Autodesk Inventor part; units mm, degrees
ref_plane "YZ Plane" through (0, 0, 0) normal (1, 0, 0) x (0, 1, 0)
ref_plane "XZ Plane" through (0, 0, 0) normal (0, 1, 0) x (-1, 0, 0)
ref_plane "XY Plane" through (0, 0, 0) normal (0, 0, 1) x (1, 0, 0)
sketch "Sketch1" plane through (0, 0, 0) normal (0, 0, 1) x (1, 0, 0)
  line L0 (6.35, 0) -> (25.4, 0)
  line L1 (25.4, 0) -> (25.4, -3.175)
  line L2 (25.4, -3.175) -> (6.35, -3.175)
  line L3 (3.175, -6.35) -> (3.175, -38.1)
  line L4 (3.175, -38.1) -> (0, -38.1)
  line L5 (0, -38.1) -> (0, -6.35)
  arc A0 (6.35, -3.175) -> (3.175, -6.35) centre (6.35, -6.35) ccw
  arc A1 (6.35, 0) -> (0, -6.35) centre (6.35, -6.35) ccw
  point P0 (0, 0)
  dimension "d0" = 3.175
  dimension "d1" = 38.1
  dimension "d2" = 3.175
  dimension "d3" = 6.35
  dimension "d6" = 25.4
extrude "Extrusion1" add sketch "Sketch1" along normal blind 50.8
hole "Hole1" at (12.7, -3.175, 38.1) direction (0, 1, 0) diameter 4.826 depth 25.4 tip angle 118
pattern_linear "Rectangular Pattern1" count 2 spacing 25 along (0, 0, -1) of "Hole1"
hole "Hole2" at (3.175, -19.05, 38.1) direction (-1, 0, 0) diameter 4.826 depth 25.4 tip angle 118
pattern_linear "Rectangular Pattern2" count 2 spacing 25.4 along (0, 0, -1) of "Hole2"
properties part number "GE-12061"
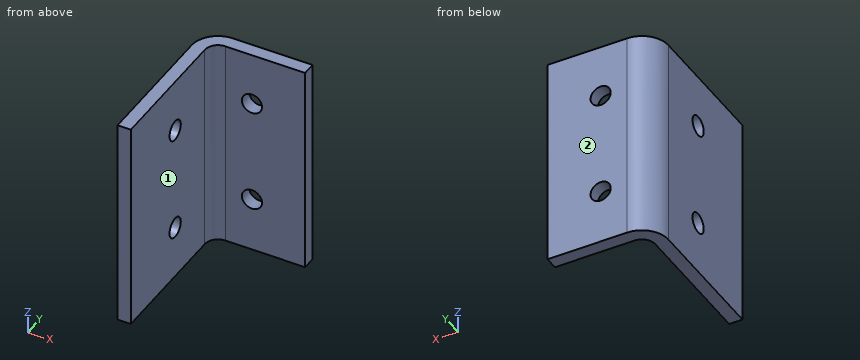
Geometry: final body of the model. Coordinates: model frame, mm. Face numbers are marked on the shaded views. A direction names the side the tool comes from. Coordinates: 2 decimals unless noted, no trailing zeros. Order: outer loops, then holes, each group sorted by start corner. A loop starts at its lowest first (then second) coordinate and runs counter-clockwise, first axis right, second up.
(1) Section query B-B (z = 38.1). Return the cut outline in (x, y) (3 decimals), plus the area to 3 significant figures.
(2) Section query D-D (z = 48). Return the cut outline in (x, y) (3 decimals).
(3) Access query for the marked faces 1 and 2. Directions: +Z, -Z, +X, -X, +Y, -Y. A direction counts if a zero-diameter tool reaches every point of the face in a straight line with its end or side. Return the directions, or none.
(4) Material intervals for probe 1 along Z at (x, y) = (1.35, -19.05); probe 2 along Z at (x, y) = (12.7, -2.15); probe 3 along Y at (x, z) = (12.75, 4.5) (3 decimals), sorted ascending.
(5) First-contact query: pin 1 (12 mm diameter, centred on x = 11, z = 20.5, fed in from -Y); pin 2 (4 mm diameter, centred on x = 12.7, z = 38.1, fed in from -Y); pin 3 (2 mm diameter, centred on y = -21.5, z = 10.5, fed in from +X) (3 decimals); pin 4 (15 mm diameter, centred on x = 19, z = 25.5, fed in from -Y) (3 decimals). Flat tips, straight axial feed; report the tip coordinate or a pass-through.
(6) Section query C-C (x = 12.7). Return the cut outline in (y, z) (3 decimals), plus the area to 3 significant figures.
(7) Section query A-A (y = -19.05). Return the cut outline in (x, z) (3 decimals), plus the area to 3 significant figures.
Solution:
1. outline: (0, -38.1) - (3.175, -38.1) - (3.175, -21.463) - (0, -21.463) - close; (0, -16.637) - (3.175, -16.637) - (3.175, -6.35) arc R3.175 cw to (6.35, -3.175) - (10.287, -3.175) - (10.287, 0) - (6.35, 0) arc R6.35 ccw to (0, -6.35) - close; (15.113, -3.175) - (25.4, -3.175) - (25.4, 0) - (15.113, 0) - close
1. area: 154 mm2
2. outline: (0, -38.1) - (3.175, -38.1) - (3.175, -6.35) arc R3.175 cw to (6.35, -3.175) - (25.4, -3.175) - (25.4, 0) - (6.35, 0) arc R6.35 ccw to (0, -6.35) - close
3. face 1: +Z, -Z, +X, -Y
3. face 2: +Z, -Z, +X, -X, +Y
4. probe 1: z = 0 to 10.29, 15.11 to 35.69, 40.51 to 50.8
4. probe 2: z = 0 to 10.69, 15.51 to 35.69, 40.51 to 50.8
4. probe 3: y = -3.175 to 0
5. pin 1: stops at y = -3.48
5. pin 2: passes through
5. pin 3: stops at x = 3.175
5. pin 4: stops at y = -3.175
6. outline: (-3.175, 0) - (0, 0) - (0, 10.687) - (-3.175, 10.687) - close; (-3.175, 15.513) - (0, 15.513) - (0, 35.687) - (-3.175, 35.687) - close; (-3.175, 40.513) - (0, 40.513) - (0, 50.8) - (-3.175, 50.8) - close
6. area: 131 mm2
7. outline: (0, 0) - (3.175, 0) - (3.175, 10.287) - (0, 10.287) - close; (0, 15.113) - (3.175, 15.113) - (3.175, 35.687) - (0, 35.687) - close; (0, 40.513) - (3.175, 40.513) - (3.175, 50.8) - (0, 50.8) - close
7. area: 131 mm2
